Geometry: see drawing. Coordinates: mm, zero at the bounding-box minimum. A direction names the side the tool comes from. Coordinates: 2 decimals unless noted, no trailing zeros. Write each loop counter-clockwise with the first axis right and the second up, starting at its lowest first coordinate (ties: lowest second). Pieces come first, ordered by that corner, then holes.
1) Set-up query: the marked faces 1 and 2. Return all of +Z, -Z, +X, -X, +Y, -Y with unobstructed straight access to the full face (end or side cutting, diameter ignored); none if empty.
2) Line query: L1, parallel to X at y = 31, z = 20; L2, parallel to Z at x = 11.75, y = 15; L3, parallel to Y at x = 20, z = 29. Output: solid intervals per line, ascending.
3) Section query C-C (x = 18.5). Output: boundary loops of the cut face in (y, z).
4) Section query B-B (y = 35.5). Output: boundary loops of the cut face in (x, z), then the cut area to 3 significant figures.
5) Section query D-D (z = 25). Output: boundary loops of the cut face in (x, y).
6) Section query A-A (z = 3). Output: boundary loops of the cut face in (x, y), then the cut area to 3 significant figures.
7) Pin query (flat end, axial travel): pin 1 Ø4 at (y, z) = (21.5, 21.5) entering from -X; pin 2 Ø4 at (x, z) = (18.5, 16.5) entering from -Y; pin 3 Ø5 at (x, y) = (11, 32.5) entering from +Z. Return the tip coordinate at first contact, or that it passes through.
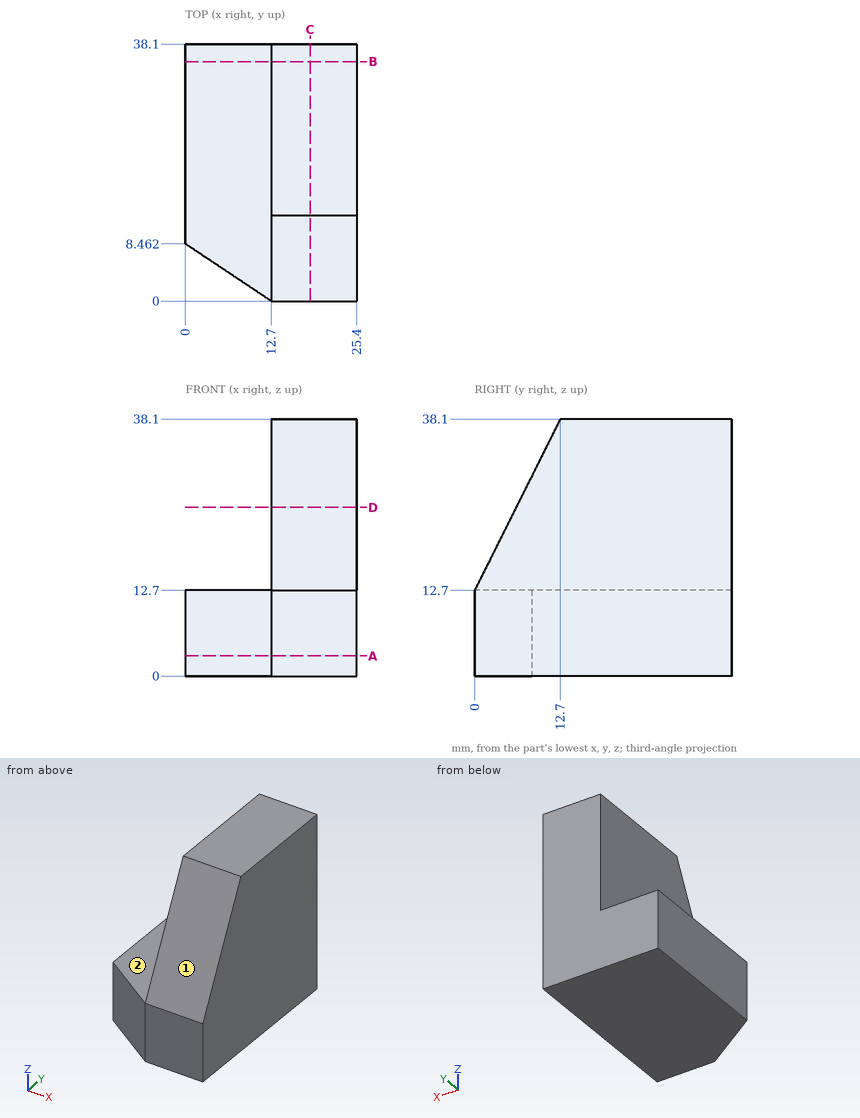
Answer:
1. face 1: +Z, +X, -X, -Y
1. face 2: +Z, -X, +Y, -Y
2. L1: x = 12.7 to 25.4
2. L2: z = 0 to 12.7
2. L3: y = 8.15 to 38.1
3. outline: (0, 0) - (38.1, 0) - (38.1, 38.1) - (12.7, 38.1) - (0, 12.7) - close
4. outline: (0, 0) - (25.4, 0) - (25.4, 38.1) - (12.7, 38.1) - (12.7, 12.7) - (0, 12.7) - close
4. area: 645 mm2
5. outline: (12.7, 6.15) - (25.4, 6.15) - (25.4, 38.1) - (12.7, 38.1) - close
6. outline: (0, 8.46) - (12.7, 0) - (25.4, 0) - (25.4, 38.1) - (0, 38.1) - close
6. area: 914 mm2
7. pin 1: stops at x = 12.7
7. pin 2: stops at y = 0.9
7. pin 3: stops at z = 38.1
